Read the model definition and answer for the solid it produces. Units are mm, in the model's axes. A direction names the side the tool comes from. Give positions to 0.01 mm unless a question says otherwise; leave off trailing zeros. Order: outer loops, then holes, each group sorted by start corner. A loop starts at its lowest first (then second) coordinate and runs counter-clockwise, first axis right, second up. Notation, with made-up numbers: (5.25, 56.5) - (63.25, 56.5) arc R28 ccw to (63.25, 79.5) - close; hole circle Ø2 at (64.5, -30). An arc over 180 degrees is marked (long way). Write item = value, one per line.
```python
from build123d import *

# Parameters (mm, degrees)
SKETCH_1_R          = 3.25
EXTRUDE_1_DEPTH     = 19.5
SKETCH_2_W          = 14
SKETCH_2_H          = 20
EXTRUDE_2_DEPTH     = 2
EXTRUDE_3_DEPTH     = 14
FILLET_1_R          = 2
EXTRUDE_4_DEPTH     = 2.5
SKETCH_6_W          = 2
SKETCH_6_H          = 2
CUT_EXTRUDE_1_DEPTH = 13.75
SKETCH_7_W          = 14
SKETCH_7_H          = 10
CUT_EXTRUDE_2_DEPTH = 2
SKETCH_8_W          = 2
SKETCH_8_H          = 2
CUT_EXTRUDE_3_DEPTH = 2.5
SKETCH_14_R         = 1.4
CUT_EXTRUDE_4_DEPTH = 2.5


with BuildPart() as part:
    # Sketch 1 → Extrude 1 (new body)
    with BuildSketch(Plane.XY):
        Circle(SKETCH_1_R)
    extrude(amount=EXTRUDE_1_DEPTH)



with BuildPart() as body_2:
    # Sketch 2 → Extrude 2 (new body)
    with BuildSketch(Plane(origin=(5, 0, 0), x_dir=(0, 0, -1), z_dir=(1, 0, 0))):
        with Locations((-9.75, 0)):
            Rectangle(SKETCH_2_W, SKETCH_2_H)
    extrude(amount=EXTRUDE_2_DEPTH)


with BuildPart() as part_1:
    add(part.part)

    add(body_2.part)  # Extrude 3 merges body 2
    # Sketch 3 → Extrude 3 (add)
    with BuildSketch(Plane(origin=(0, 0, 2.75), x_dir=(-1, 0, 0), z_dir=(0, 0, -1))):
        Polygon((0, 0), (-5, 4.5), (-5, -4.5), align=None)
    extrude(amount=-EXTRUDE_3_DEPTH)

    # Fillet 1
    fillet_1_edges = [part_1.edges().sort_by_distance(p)[0] for p in [
        (2.415705975, 2.174135378, 9.75),
        (2.415705975, -2.174135378, 9.75),
        (5, 4.5, 9.75),
        (5, -4.5, 9.75),
    ]]
    fillet(fillet_1_edges, radius=FILLET_1_R)

    # Sketch 5 → Extrude 4 (add)
    with BuildSketch(Plane(origin=(7, 0, 0), x_dir=(0, 0, -1), z_dir=(1, 0, 0))):
        Polygon((-21.297005384, 20), (-32.844010768, 0), (-21.297005384, -20), (1.797005384, -20), (13.344010768, 0), (1.797005384, 20), align=None)
    extrude(amount=EXTRUDE_4_DEPTH)

    # Sketch 6 → Cut-Extrude 1 (cut, through all)
    with BuildSketch(Plane(origin=(9.5, 0, 0), x_dir=(0, 0, -1), z_dir=(1, 0, 0))):
        with Locations((-13, 0)):
            Rectangle(SKETCH_6_W, SKETCH_6_H)
        with Locations((-6.5, 0)):
            Rectangle(SKETCH_6_W, SKETCH_6_H)
    extrude(amount=-CUT_EXTRUDE_1_DEPTH, mode=Mode.SUBTRACT)

    # Sketch 7 → Cut-Extrude 2 (cut)
    with BuildSketch(Plane(origin=(9.5, 0, 0), x_dir=(0, 0, -1), z_dir=(1, 0, 0))):
        with Locations((-9.75, 0)):
            Rectangle(SKETCH_7_W, SKETCH_7_H)
    extrude(amount=-CUT_EXTRUDE_2_DEPTH, mode=Mode.SUBTRACT)

    # Sketch 8 → Cut-Extrude 3 (cut)
    with BuildSketch(Plane(origin=(9.5, 0, 0), x_dir=(0, 0, -1), z_dir=(1, 0, 0))):
        with Locations((-17.75, 0)):
            Rectangle(SKETCH_8_W, SKETCH_8_H)
        with Locations((-1.75, 0)):
            Rectangle(SKETCH_8_W, SKETCH_8_H)
    extrude(amount=-CUT_EXTRUDE_3_DEPTH, mode=Mode.SUBTRACT)

    # Sketch 14 → Cut-Extrude 4 (cut)
    with BuildSketch(Plane(origin=(9.5, 0, 0), x_dir=(0, 0, -1), z_dir=(1, 0, 0))):
        with Locations((-9.75, 15)):
            Circle(SKETCH_14_R)
        with Locations((3.240381057, 7.5)):
            Circle(SKETCH_14_R)
        with Locations((3.240381057, -7.5)):
            Circle(SKETCH_14_R)
        with Locations((-9.75, -15)):
            Circle(SKETCH_14_R)
        with Locations((-22.740381057, -7.5)):
            Circle(SKETCH_14_R)
        with Locations((-22.740381057, 7.5)):
            Circle(SKETCH_14_R)
    extrude(amount=-CUT_EXTRUDE_4_DEPTH, mode=Mode.SUBTRACT)


solid = part_1.part
```
1. Section B-B (y = 7.5) is taken. Determine the outline of the cut face in (x, z).
Recorded:
outline = (5, 2.75) - (7, 2.75) - (7, -1.84) - (9.5, -1.84) - (9.5, 21.34) - (7, 21.34) - (7, 16.75) - (5, 16.75) - close; (7, -9.01) - (9.5, -9.01) - (9.5, -4.64) - (7, -4.64) - close; (7, 24.14) - (9.5, 24.14) - (9.5, 28.51) - (7, 28.51) - close
2. Section A-A (x = 0) is taken. Determine the outline of the cut face in (y, z), and give its area (3 significant figures).
Recorded:
outline = (-3.25, 0) - (3.25, 0) - (3.25, 19.5) - (-3.25, 19.5) - close; hole (-1, 5.5) - (1, 5.5) - (1, 7.5) - (-1, 7.5) - close; hole (-1, 12) - (1, 12) - (1, 14) - (-1, 14) - close
area = 119 mm^2
3. Determine the mould class of faces 1 (the face through (8.23, -9.86, 27.15)), 2 (the face through (8, -20, 10)), 3 (the face through (2, -1, 13)) for opening direction Z: +Z half, -Z half, draft (parallel to the pull), parting line (faces both ways), or undercut.
Recorded:
face_1 = +Z half
face_2 = draft
face_3 = undercut
4. Flat-ended cylindrical pins translate along their axes: pin 1 (4.5 mm diameter, centred on y = 7.5, z = -3.24, fed in from -X); pin 2 (0.6 mm diameter, centred on x = 6, z = 11.5, fed in from -Y); pin 3 (0.6 mm diameter, centred on x = 4, y = 0, fed in from -Z); pin 4 (2 mm diameter, centred on y = -15, z = 9.75, fed in from -X). Find the tip coordinate at first contact, or state that the pin passes through.
Recorded:
pin_1 = 7
pin_2 = -10
pin_3 = 2.75
pin_4 = through
5. Straight lines are drawn through the part: L1, parallel to Z at x = 2.25, y = 0.5; L2, parallel to Y at x = 8, z = 9.75; L3, parallel to Z at x = 4.75, y = 4. For each, find the intervals that lie inside material, in ascending order. Write a range as [from, to].
Recorded:
L1 = [0, 5.5], [7.5, 12], [14, 19.5]
L2 = [-20, -16.4], [-13.6, -5], [5, 13.6], [16.4, 20]
L3 = [2.75, 16.75]
6. Section C-C (z = 20.5) is taken. Determine the outline of the cut face in (x, y).
Recorded:
outline = (7, -20) - (9.5, -20) - (9.5, 20) - (7, 20) - close
7. Section D-D (y = -2) is taken. Determine the outline of the cut face in (x, z), and give its area (3 significant figures).
Recorded:
outline = (-2.56, 0) - (2.56, 0) - (2.56, 2.75) - (7, 2.75) - (7, -12.19) - (9.5, -12.19) - (9.5, 2.75) - (7.5, 2.75) - (7.5, 16.75) - (9.5, 16.75) - (9.5, 31.69) - (7, 31.69) - (7, 16.75) - (2.56, 16.75) - (2.56, 19.5) - (-2.56, 19.5) - close
area = 244 mm^2
8. For faces 4 (the face through (4.822, -4.566, 9.848)), 5 (the face through (9, 5, 10)), 6 (the face through (2, 0, 12)), determine the directions among +Z, -Z, +X, -X, +Y, -Y from which every point of the face is accessible in a straight line to the end or side of a thin tool.
Recorded:
face_4 = +Z, -Z, -X, -Y
face_5 = +X
face_6 = +X, -X
